```python
from build123d import *

# Parameters (mm, degrees)
SKETCH1_W           = 26.5
SKETCH1_H           = 47.5
SKETCH1_W_2         = 21.5
SKETCH1_H_2         = 42.5
BOSS_EXTRUDE1_DEPTH = 33
SKETCH2_W           = 21.5
SKETCH2_H           = 42.5
BOSS_EXTRUDE2_DEPTH = 2.5
CUT_EXTRUDE2_DEPTH  = 2.5
SKETCH4_W           = 9.75
SKETCH4_H           = 8
SKETCH4_W_2         = 26.5
BOSS_EXTRUDE3_DEPTH = 2.5
SKETCH7_W           = 47.5
SKETCH7_H           = 30.5
BOSS_EXTRUDE5_DEPTH = 20
SKETCH8_W           = 47.5
SKETCH8_H           = 10
BOSS_EXTRUDE6_DEPTH = 2.5
SKETCH9_R           = 1.5
CUT_EXTRUDE3_DEPTH  = 21.5


with BuildPart() as part:
    # Sketch1 → Boss-Extrude1 (new body)
    with BuildSketch(Plane(origin=(0, 0, 0), x_dir=(1, 0, 0), z_dir=(0, 1, 0))):
        with Locations((0.956397274, -2.454043299)):
            Rectangle(SKETCH1_W, SKETCH1_H)
        with Locations((0.956397274, -2.454043299)):
            Rectangle(SKETCH1_W_2, SKETCH1_H_2, mode=Mode.SUBTRACT)
    extrude(amount=BOSS_EXTRUDE1_DEPTH)

    # Sketch2 → Boss-Extrude2 (add)
    with BuildSketch(Plane(origin=(0, 33, 0), x_dir=(1, 0, 0), z_dir=(0, 1, 0))):
        with Locations((0.956397274, -2.454043299)):
            Rectangle(SKETCH2_W, SKETCH2_H)
    extrude(amount=-BOSS_EXTRUDE2_DEPTH)

    # Sketch3 → Cut-Extrude2 (cut)
    with BuildSketch(Plane(origin=(0, 0, -21.295956701), x_dir=(-1, 0, 0), z_dir=(0, 0, -1))):
        Polygon((2.543602726, 30.5), (2.543602726, 0), (-0.956397274, 0), (-4.456397274, 0), (-4.456397274, 30.5), align=None)
    extrude(amount=-CUT_EXTRUDE2_DEPTH, mode=Mode.SUBTRACT)

    # Sketch4 → Boss-Extrude3 (add)
    with BuildSketch(Plane.XZ):
        with Locations((-7.418602726, -25.295956701)):
            Rectangle(SKETCH4_W, SKETCH4_H)
        with Locations((0.956397274, 30.204043299)):
            Rectangle(SKETCH4_W_2, SKETCH4_H)
        with Locations((9.331397274, -25.295956701)):
            Rectangle(SKETCH4_W, SKETCH4_H)
    extrude(amount=-BOSS_EXTRUDE3_DEPTH)

    # Sketch7 → Boss-Extrude5 (add)
    with BuildSketch(Plane(origin=(14.206397274, 0, 0), x_dir=(0, 0, -1), z_dir=(1, 0, 0))):
        with Locations((-2.454043299, 17.75)):
            Rectangle(SKETCH7_W, SKETCH7_H)
    extrude(amount=BOSS_EXTRUDE5_DEPTH)

    # Sketch8 → Boss-Extrude6 (add)
    with BuildSketch(Plane(origin=(34.206397274, 0, 0), x_dir=(0, 0, -1), z_dir=(1, 0, 0))):
        with Locations((-2.454043299, 38)):
            Rectangle(SKETCH8_W, SKETCH8_H)
        with Locations((-2.454043299, -2.5)):
            Rectangle(SKETCH8_W, SKETCH8_H)
    extrude(amount=-BOSS_EXTRUDE6_DEPTH)

    # Sketch9 → Cut-Extrude3 (cut)
    with BuildSketch(Plane.ZY.offset(-31.706397274)):
        with Locations((-7.545956701, -3.75)):
            Circle(SKETCH9_R)
        with Locations((12.454043299, -3.75)):
            Circle(SKETCH9_R)
        with Locations((-7.545956701, 38)):
            Circle(SKETCH9_R)
        with Locations((12.454043299, 38)):
            Circle(SKETCH9_R)
    extrude(amount=-CUT_EXTRUDE3_DEPTH, mode=Mode.SUBTRACT)


solid = part.part
```
Can you work these out from the model? Positions are in its coordinate system, mm. A direction names the side the tool comes from. Round coordinates to 2 decimals unless told otherwise and drop trailing zeros. Loops run counter-clockwise (first coordinate to the right, second up) from the corner with the lowest first, then second, coordinate; pieces in that order, holes last.
Item 1: Which directions (+Z, -Z, +X, -X, +Y, -Y) give clear straight access to the entire face, cutting with the end or side of a thin tool? Please do faces 1 (the flat face through (1, 2.5, 30)), 2 (the flat face through (14.206, 1, 3)), 3 (the flat face through (11.706, 15, 3)), 4 (the flat face through (9, 2.5, -25)).
Item 2: Please list where these lines run through material, in increasing order: L1, parallel to X at y = 26.5, z = -10.5; L2, parallel to Z at x = 10, y = 13; L3, parallel to Y at x = -8, z = 2.5.
Item 3: Suppose I cut it at D-D, the plane x = 5.5. Write out the boundary of the cut face in (y, z), then the cut area to 3 significant figures.
Item 4: Will these pins go through, and if not, where does the flat tip stop? pin 1 Ø2 at (x, y) = (-6, 9) entering from +Z; pin 2 Ø23.5 at (x, y) = (-0.5, 15) entering from -Z; pin 3 Ø2 at (x, z) = (22.5, 1) entering from +Y; pin 4 Ø11.5 at (y, z) = (19.5, -26.5) entering from -X.
Item 5: Suppose I cut it at A-A, the plane y = -3.75. Write out the boundary of the cut face in (x, z), then the cut area to 3 significant figures.
Item 6: Suppose I cut it at B-B, the plane y = 1.5. Write out the boundary of the cut face in (x, z), then the cut area to 3 significant figures.
Item 7: If we mould it in two halves opening along X, with no side actions, what happens to faces 5 (the flat face through (34.206, 18, 3)), 6 (the flat face through (23, 2.5, 3)), 7 (the flat face through (31.706, 38, 3)), 8 (the flat face through (1, 1, 34.204))? For each: +X half, -X half, draft (parallel to the pull), parting line (faces both ways), or undercut.
Item 8: Suppose I cut it at C-C, the plane z = -25. Write out the boundary of the cut face in (x, y), then the cut area to 4 significant figures.
Reported:
1. face 1: +Z, +X, -X, +Y
1. face 2: +Z, -Z, -Y
1. face 3: -Y
1. face 4: -Z, +X, -X, +Y
2. L1: x = -12.29 to -9.79, 11.71 to 34.21
2. L2: z = -21.3 to -18.8, 23.7 to 26.2
2. L3: y = 30.5 to 33
3. outline: (0, -29.3) - (2.5, -29.3) - (2.5, -21.3) - (33, -21.3) - (33, 26.2) - (2.5, 26.2) - (2.5, 34.2) - (0, 34.2) - (0, 23.7) - (30.5, 23.7) - (30.5, -18.8) - (0, -18.8) - close
3. area: 311 mm2
4. pin 1: stops at z = 26.2
4. pin 2: stops at z = -21.3
4. pin 3: stops at y = 33
4. pin 4: stops at x = -12.29
5. outline: (31.71, -21.3) - (34.21, -21.3) - (34.21, -9.05) - (31.71, -9.05) - close; (31.71, -6.05) - (34.21, -6.05) - (34.21, 10.95) - (31.71, 10.95) - close; (31.71, 13.95) - (34.21, 13.95) - (34.21, 26.2) - (31.71, 26.2) - close
5. area: 104 mm2
6. outline: (-12.29, -29.3) - (-2.54, -29.3) - (-2.54, -18.8) - (-9.79, -18.8) - (-9.79, 23.7) - (11.71, 23.7) - (11.71, -18.8) - (4.46, -18.8) - (4.46, -29.3) - (14.21, -29.3) - (14.21, 34.2) - (-12.29, 34.2) - close; (31.71, -21.3) - (34.21, -21.3) - (34.21, 26.2) - (31.71, 26.2) - close
6. area: 814 mm2
7. face 5: +X half
7. face 6: undercut
7. face 7: -X half
7. face 8: draft
8. outline: (-12.29, 0) - (-2.54, 0) - (-2.54, 2.5) - (-12.29, 2.5) - close; (4.46, 0) - (14.21, 0) - (14.21, 2.5) - (4.46, 2.5) - close
8. area: 48.75 mm2
